Verification items for this drawing (mm, ordinates from the low corner). Round coordinates to 2 decimals unless told otherwise and drop trailing zeros. Order: outer loops, then holes, each group sorted by start corner. A loop starts at its lowest first (then second) coordinate and runs counter-clockwise, first axis right, second up. Notation, with made-up numbers: (82, 45.25) -> (94, 45.25) arc R26 ccw to (94, 61.25) -> close; hole circle Ø8 at (33.25, -9.75). An arc over 180 degrees is marked (long way). Put each result on its own line as item: value.
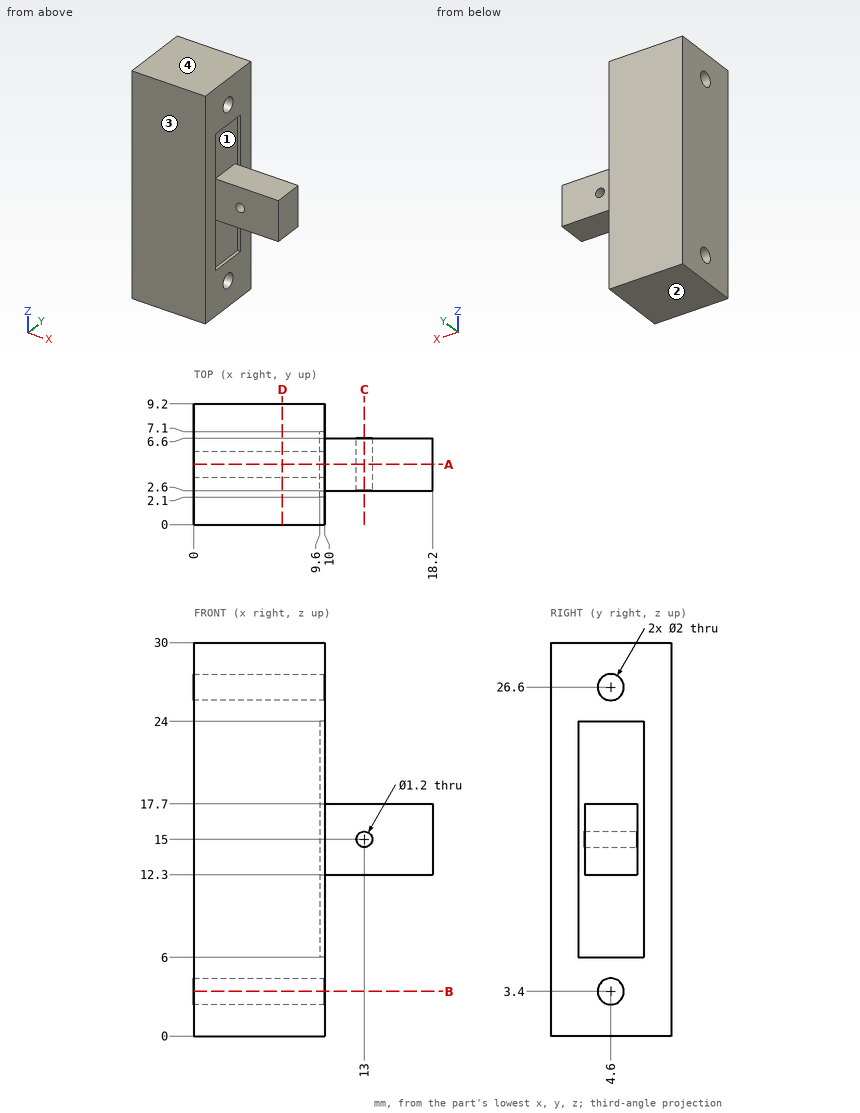
Item 1: Section check B-B on z = 3.4. Record the boundary of the cut face in (x, y).
Check sheet entries:
outline: (0, 0) -> (10, 0) -> (10, 3.6) -> (0, 3.6) -> close; (0, 5.6) -> (10, 5.6) -> (10, 9.2) -> (0, 9.2) -> close
Item 2: Release check for a two-part mould opening along Z. For the marked faces 1, 2, 3 and 4 record: +Z half, -Z half, draft (parallel to the pull), parting line (faces both ways), or undercut.
Check sheet entries:
face 1: undercut
face 2: -Z half
face 3: draft
face 4: +Z half
Item 3: Gauge pin test, flat ends, axial feed: pin 1 Ø3 at (x, z) = (2.5, 12.5) entering from -Y; pin 2 Ø6 at (x, z) = (16, 14.5) entering from -Y; pin 3 Ø1.2 at (x, y) = (15, 5.5) entering from +Z; pin 4 Ø1 at (y, z) = (3, 26.5) entering from +X. Record the tip position at first contact, or that the pin passes through.
Check sheet entries:
pin 1: stops at y = 0
pin 2: stops at y = 2.6
pin 3: stops at z = 17.7
pin 4: stops at x = 10
Item 4: Section check D-D on x = 6.75. Record the boundary of the cut face in (y, z), then the cut area to 3 significant figures.
Check sheet entries:
outline: (0, 0) -> (9.2, 0) -> (9.2, 30) -> (0, 30) -> close; hole circle Ø2 at (4.6, 3.4); hole circle Ø2 at (4.6, 26.6)
area: 270 mm^2
Item 5: Material ranges on L1, parallel to Z at x = 1, y = 4.5; L2, parallel to Y at x = 3.25, z = 3.4; L3, parallel to X at y = 5.3, z = 15, recorded low to high. Write a range as [from, to].
Check sheet entries:
L1: z = [0, 2.41], [4.39, 25.61], [27.59, 30]
L2: y = [0, 3.6], [5.6, 9.2]
L3: x = [0, 12.4], [13.6, 18.2]
Item 6: Section check A-A on y = 4.6. Record the boundary of the cut face in (x, z).
Check sheet entries:
outline: (0, 0) -> (10, 0) -> (10, 2.4) -> (0, 2.4) -> close; (0, 4.4) -> (10, 4.4) -> (10, 6) -> (9.6, 6) -> (9.6, 12.3) -> (18.2, 12.3) -> (18.2, 17.7) -> (9.6, 17.7) -> (9.6, 24) -> (10, 24) -> (10, 25.6) -> (0, 25.6) -> close; (0, 27.6) -> (10, 27.6) -> (10, 30) -> (0, 30) -> close; hole circle Ø1.2 at (13, 15)
Item 7: Section check C-C on x = 13. Record the boundary of the cut face in (y, z).
Check sheet entries:
outline: (2.6, 12.3) -> (6.6, 12.3) -> (6.6, 14.4) -> (2.6, 14.4) -> close; (2.6, 15.6) -> (6.6, 15.6) -> (6.6, 17.7) -> (2.6, 17.7) -> close
